from build123d import *

# Parameters (mm, degrees)
F0_W     = 50
F0_H     = 100
F0_W_2   = 40
F0_H_2   = 90
F1_DEPTH = 15
F2_R     = 2.5
F3_DEPTH = 50.001


with BuildPart() as f1:
    # F0 (on Front) → F1 (new body)
    with BuildSketch(Plane.XZ):
        with Locations((-0.139878, 2.446302)):
            Rectangle(F0_W, F0_H)
        with Locations((-0.139878, 2.446302)):
            Rectangle(F0_W_2, F0_H_2, mode=Mode.SUBTRACT)
    extrude(amount=F1_DEPTH)

    # F2 (on face) → F3 (cut, through all)
    with BuildSketch(Plane(origin=(-25.139878, 0, 0), x_dir=(0, -1, 0), z_dir=(-1, 0, 0))):
        with Locations((7.5, 30)):
            Circle(F2_R)
        with Locations((7.5, 0)):
            Circle(F2_R)
        with Locations((7.5, -30)):
            Circle(F2_R)
    extrude(amount=-F3_DEPTH, mode=Mode.SUBTRACT)


solid = f1.part
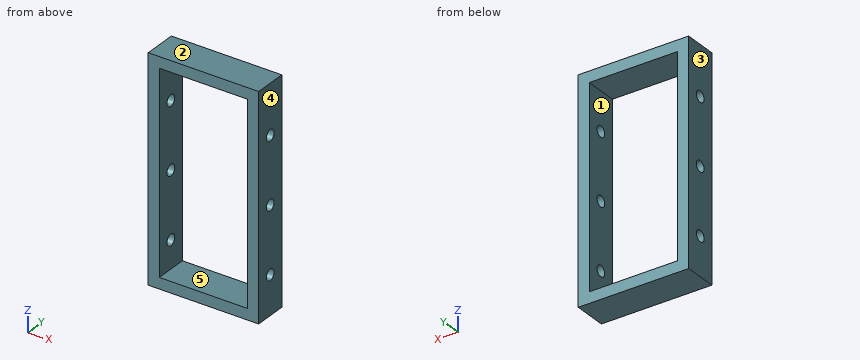
For this review, take the finished solid that the model builds, in its own axes (mm). Face numbers are marked on the shaded views. A direction names the side the tool comes from. Give positions to 0.01 mm unless a question says otherwise; leave off trailing zeros. Loops run counter-clockwise (first coordinate to the right, second up) from the corner with the lowest first, then second, coordinate; pieces in that order, holes last. Notation, with made-up numbers: (70, 41) -> (124, 41) arc R12 ccw to (124, 54) -> close; hole circle Ø1 at (-33, 14.5). An arc over 180 degrees is marked (long way). One line per question, with ' | ' between items.
1) We need section D-D (y = -2). Write out the cut boundary in (x, z).
Resolved:
outline: (-25.14, -47.55) -> (24.86, -47.55) -> (24.86, 52.45) -> (-25.14, 52.45) -> close; hole (-20.14, -42.55) -> (19.86, -42.55) -> (19.86, 47.45) -> (-20.14, 47.45) -> close
2) We need section C-C (x = -8.5). Write out the cut boundary in (y, z), plus the area to 3 significant figures.
Resolved:
outline: (-15, -47.55) -> (0, -47.55) -> (0, -42.55) -> (-15, -42.55) -> close; (-15, 47.45) -> (0, 47.45) -> (0, 52.45) -> (-15, 52.45) -> close | area: 150 mm2
3) For the marked faces 4 and 5, list the 3-axis set-ups (+Z, -Z, +X, -X, +Y, -Y) from which the entire face can be reached by the end or side of a thin tool; tool diameter is ignored.
Resolved:
face 4: +Z, -Z, +X, +Y, -Y | face 5: +Y, -Y
4) We need section B-B (z = 19.5). Write out the cut boundary in (x, y), plus the area to 3 significant figures.
Resolved:
outline: (-25.14, -15) -> (-20.14, -15) -> (-20.14, 0) -> (-25.14, 0) -> close; (19.86, -15) -> (24.86, -15) -> (24.86, 0) -> (19.86, 0) -> close | area: 150 mm2
5) Insertion check: pin 1 Ø3 at (y, z) = (-7.5, 30) entering from -X; pin 2 Ø10 at (x, z) = (-19.5, -33) entering from +Y. Each pin has a flat end and moves straight along its axis. Give the tip position at first contact, or say it passes through.
Resolved:
pin 1: passes through | pin 2: stops at y = 0
6) We need section A-A (y = -7.5). Give the number of separate pieces and of enclosed holes in the cut face, plus the area to 3 significant figures.
Resolved:
separate pieces: 6 | enclosed holes: 0 | area: 1,250 mm2
7) To check wall thickness, follow probe 1 along Z at (x, y) = (-23.6, -7.5); probe 2 along X at (y, z) = (-2.25, 11); probe 3 along Z at (x, y) = (-12.5, -12.5). State the ranges of each line that lie inside material, in increasing order.
Resolved:
probe 1: z = -47.55 to -32.5, -27.5 to -2.5, 2.5 to 27.5, 32.5 to 52.45 | probe 2: x = -25.14 to -20.14, 19.86 to 24.86 | probe 3: z = -47.55 to -42.55, 47.45 to 52.45
8) The part is to be moulded in two halves that separate along Z. For the marked faces 1, 2 and 3, say which applies: +Z half, -Z half, draft (parallel to the pull), parting line (faces both ways), or undercut.
Resolved:
face 1: undercut | face 2: +Z half | face 3: draft
